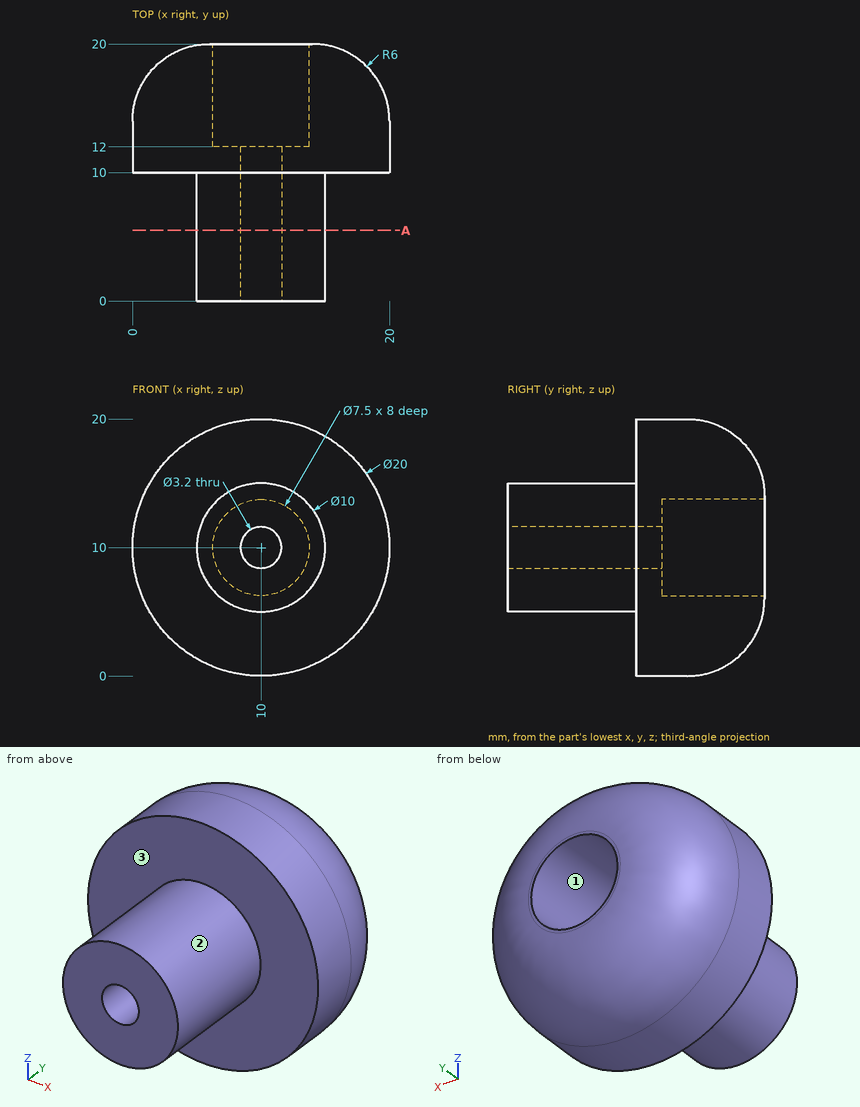
Verification items for this drawing (mm, ordinates from the low corner). Coordinates: 2 decimals unless noted, no trailing zeros. Write each loop counter-clockwise with the first axis right and the second up, starting at its lowest first coordinate (ties: lowest second). Pieces come first, ordered by that corner, then holes. Notation, with made-up numbers: M 5.5,39.5 L 46.5,39.5 A23 cw 46.5,67.5 Z; hole C -40,-26.5 d11. An arc over 180 degrees is marked long. Answer as a JSON object with one key per item and string values. Group by question number.
(1) Gauge pin test, flat ends, axial feed: pin 1 (1.5 mm diameter, centred on y = 7.5, z = 2.5, fed in from -X); pin 2 (10 mm diameter, centred on x = 17.5, y = 15.5, fed in from +Z); pin 3 (1 mm diameter, centred on y = 5.5, z = 14.5, fed in from -X); pin 4 (1 mm diameter, centred on y = 14.5, z = 14, fed in from -X). Record the tip position at first contact, or that the pin passes through.
(2) Cross-section at A-A, the plane y = 5.5. Record the cut outline in (x, z), and give its area (3 significant figures).
(3) Material ranges on line 1 (X direction, y = 7, z = 10); line 2 (Y direction, x = 7, z = 12.75); line 3 (X direction, y = 7.75, z = 9.25), recorded low to high.
(4) Release check for a two-part mould opening along X. For the marked faces 1, 2 and 3 record: +X half, -X half, draft (parallel to the pull), parting line (faces both ways), or undercut.
Reply:
{
 "1": {"pin 1": "through", "pin 2": "z = 19.64", "pin 3": "x = 7", "pin 4": "x = 0.65"},
 "2": {"outline": "C 10,10 d10; hole C 10,10 d3.2", "area": "70.5 mm²"},
 "3": {"line 1": "5 to 8.4, 11.6 to 15", "line 2": "0 to 20", "line 3": "5.06 to 8.59, 11.41 to 14.94"},
 "4": {"face 1": "undercut", "face 2": "parting line", "face 3": "draft"}
}
